```python
from build123d import *

# Parameters (mm, degrees)
F1_DEPTH  = 48.26
F2_R      = 6.35
F3_DEPTH  = 20.066
F4_W      = 90.932
F4_H      = 26.7915036529
F5_DEPTH  = 63.5
F6_W      = 12.1428427496
F6_H      = 35.56
F7_DEPTH  = 70.866
F8_W      = 35.7905875854
F8_H      = 25.4
F9_DEPTH  = 10.16
F11_START = 10.414
F10_W     = 19.304
F10_H     = 47.7508436888
F11_DEPTH = 11.176


with BuildPart() as f1:
    # F0 (on Top) → F1 (new body)
    with BuildSketch(Plane.XY):
        Polygon((59.8277186039, -32.457854175), (59.8277186039, 28.502145825), (31.3797186039, 28.502145825), (31.3797186039, 15.802145825), (-28.7564180376, 15.802145825), (-59.5522813961, -1.977854175), (-28.7564180376, -19.757854175), (31.3797186039, -19.757854175), (31.3797186039, -32.457854175), align=None)
    extrude(amount=F1_DEPTH)

    # F2 (on Front) → F3 (cut, symmetric)
    with BuildSketch(Plane.XZ):
        with Locations((-3.6722813961, 12.7)):
            Circle(F2_R)
    extrude(amount=F3_DEPTH, both=True, mode=Mode.SUBTRACT)

    # F4 (on Front) → F5 (cut, symmetric)
    with BuildSketch(Plane.XZ):
        with Locations((-14.0862813961, 34.9018583074)):
            Rectangle(F4_W, F4_H)
    extrude(amount=F5_DEPTH, both=True, mode=Mode.SUBTRACT)

    # F6 (on Top) → F7 (cut)
    with BuildSketch(Plane.XY):
        with Locations((54.0386456996, -1.977854175)):
            Rectangle(F6_W, F6_H)
    extrude(amount=F7_DEPTH, mode=Mode.SUBTRACT)

    # F8 (on face) → F9 (cut)
    with BuildSketch(Plane.XY.offset(48.26)):
        with Locations((38.911470212, -1.977854175)):
            Rectangle(F8_W, F8_H)
    extrude(amount=-F9_DEPTH, mode=Mode.SUBTRACT)

    # F10 (on Top) → F11 (cut)
    with BuildSketch(Plane.XY.offset(F11_START)):
        with Locations((-49.9002813961, -3.6451024935)):
            Rectangle(F10_W, F10_H)
    extrude(amount=F11_DEPTH, mode=Mode.SUBTRACT)


solid = f1.part
```
Design review of the part built by this model. Coordinates are the model's own, in mm. A direction names the side the tool comes from. Give positions to 0.01 mm unless a question says otherwise; leave off trailing zeros. Loops run counter-clockwise (first coordinate to the right, second up) from the corner with the lowest first, then second, coordinate; pieces in that order, holes last. Notation, with made-up numbers: M 56.5,-22 L 64.5,-22 A23 cw 64.5,16 Z; hole C -2,53 d8. An arc over 180 degrees is marked long. Return JSON: item names as keys, results as strings. Group by question number.
Item 1: Tool access review of faces 4 (the flat face through (2, 15.802, 8)), 5 (the flat face through (-40.248, -2, 16)), 6 (the flat face through (1, -19.758, 8)), 7 (the flat face through (54, 15.802, 24)): name each direction out of +Z, -Z, +X, -X, +Y, -Y from which nothing blocks a thin tool from reaching the whole face with its end or side.
Item 2: We need section D-D (z = 5). Give the boundary of the cut face in (x, y).
Item 3: Insertion check: pin 1 Ø1.5 at (x, y) = (-28, 16) entering from +Z; pin 2 Ø1 at (y, z) = (-7.5, 20.5) entering from +X; pin 3 Ø11 at (x, z) = (-4, 10) entering from +Y. Each pin has a flat end and moves straight along its axis. Give the tip position at first contact, or say it passes through.
Item 4: Mouldability with a two-part tool opening along Z and no side actions: class faces 1 (the flat face through (-40.95, -12.72, 8.21)), 2 (the cylindrical face through (-4.499, -2.227, 18.996)), 3 (the flat face through (40, -2, 38.1)) as released by +Z, released by -Z, zero draft, split by the parting line, or undercut.
Item 5: For probe 1 along X at (y, z) = (24, 35); probe 2 along X at (y, z) = (-10, 20); probe 3 along Y at (x, z) = (51.5, 21), list the stretches that pass through material, from the lowest coordinate up.
Item 6: We need section A-A (z = 12.7). Give the boundary of the cut face in (x, y), and give its area (3 significant figures).
Item 7: We need section B-B (x = 43.5). Give the boundary of the cut face in (y, z), and give its area (3 significant figures).
Item 8: We need section C-C (y = 14). Give the boundary of the cut face in (x, z).
Output:
{
 "1": {"face 4": "+Z, -Z, -X, +Y", "face 5": "+Z, -X, +Y, -Y", "face 6": "+Z, -Z, -X, -Y", "face 7": "+Z, -Z, +X"},
 "2": {"outline": "M -59.55,-1.98 L -28.76,-19.76 L 31.38,-19.76 L 31.38,-32.46 L 59.83,-32.46 L 59.83,-19.76 L 47.97,-19.76 L 47.97,15.8 L 59.83,15.8 L 59.83,28.5 L 31.38,28.5 L 31.38,15.8 L -28.76,15.8 Z"},
 "3": {"pin 1": "stops at z = 21.51", "pin 2": "stops at x = 47.97", "pin 3": "stops at y = 15.8"},
 "4": {"face 1": "zero draft", "face 2": "undercut", "face 3": "released by +Z"},
 "5": {"probe 1": "x = 31.38 to 59.83", "probe 2": "x = -40.25 to 47.97", "probe 3": "y = -32.46 to -19.76, 15.8 to 28.5"},
 "6": {"outline": "M -40.25,-13.12 L -28.76,-19.76 L -10.02,-19.76 L -10.02,15.8 L -28.76,15.8 L -40.25,9.17 Z; M 2.68,-19.76 L 31.38,-19.76 L 31.38,-32.46 L 59.83,-32.46 L 59.83,-19.76 L 47.97,-19.76 L 47.97,15.8 L 59.83,15.8 L 59.83,28.5 L 31.38,28.5 L 31.38,15.8 L 2.68,15.8 Z", "area": "3,330 mm^2"},
 "7": {"outline": "M -32.46,0 L 28.5,0 L 28.5,48.26 L 10.72,48.26 L 10.72,38.1 L -14.68,38.1 L -14.68,48.26 L -32.46,48.26 Z", "area": "2,680 mm^2"},
 "8": {"outline": "M -31.88,0 L 47.97,0 L 47.97,48.26 L 31.38,48.26 L 31.38,21.51 L -31.88,21.51 Z; hole C -3.67,12.7 d12.7"}
}
